Build history of the part. All positions in model axes, mm. Face numbers are marked on the shaded views. A direction names the side the tool comes from. Give positions to 0.01 mm unless a question says otherwise; leave off trailing zeros. Loops run counter-clockwise (first coordinate to the right, second up) from the corner with the lowest first, then second, coordinate; pieces in that order, holes last. Notation, with made-up numbers: (83.25, -5.5) -> (97.25, -5.5) arc R12 ccw to (97.25, -0.5) -> close; hole circle Ø7 at (76.25, 42.25). An arc over 180 degrees is marked (long way). One line per question, with ' | ' between items. Start each with the question number.
(1) Slice it at C-C, the plane y = -28.5. Write the cut outline in (x, z).
(2) Flat gauge pins, fed straight in: pin 1 Ø10 at (x, y) = (15.748, -38.1) entering from -Z; pin 2 Ø12 at (y, z) = (-36, -13.5) entering from -X; pin 3 Ø5 at (x, y) = (110.5, -44) entering from +Z. Where does each tip first touch, or does it go through?
(3) Slice it at D-D, the plane x = 95. Write the cut outline in (y, z).
(4) 3-axis set-ups, long thin cutter, end or side, ignore diameter. For the marked faces 1 and 2: which of +Z, -Z, +X, -X, +Y, -Y reach the whole face in a straight line?
(5) Slice it at A-A, the plane y = -38.1. Write the cut outline in (x, z) (1 decimal).
(6) Drill centre lines: L1, parallel to X at y = -38.1, z = 9.5 (3 decimals); L2, parallel to X at y = -38.1, z = 4.5; L3, parallel to Y at x = 114, z = 4.5. Where is each one in solid material? Low to high. Write a range as from..to.
(7) Slice it at B-B, the plane x = 58. Write the cut outline in (y, z).
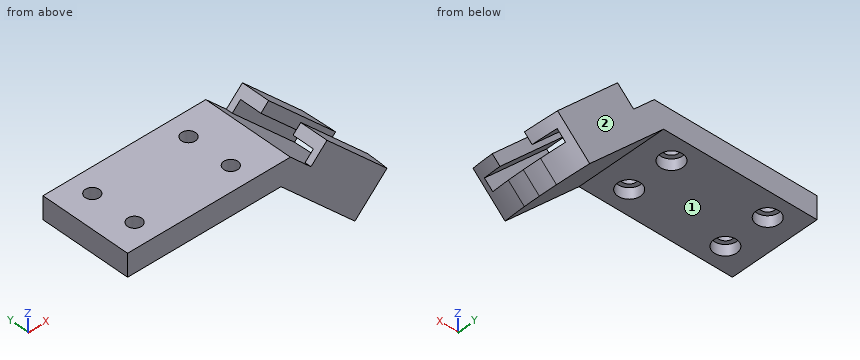
```python
from build123d import *

# Parameters (mm, degrees)
F1_DEPTH       = 50.8
F3_D           = 7.874
F3_CBORE_D     = 12.7
F3_CBORE_DEPTH = 6.096
F4_D           = 7.874
F4_CBORE_D     = 12.7
F4_CBORE_DEPTH = 6.096
F6_DEPTH       = 53.848
F8_DEPTH       = 53.848
F10_DEPTH      = 25.4


with BuildPart() as f1:
    # F0 (on Front) → F1 (new body)
    with BuildSketch(Plane.XZ):
        Polygon((0, 12.7), (0, 0), (85.852, 0), (131.70327, -45.85127), (140.683526, -36.871014), (91.112512, 12.7), align=None)
    extrude(amount=F1_DEPTH)

    # F3 (through all)
    with Locations(Plane(origin=(0, 0, 0), x_dir=(1, 0, 0), z_dir=(0, 0, -1))):
        with Locations((15.748, 38.1)):
            CounterBoreHole(F3_D / 2, F3_CBORE_D / 2, F3_CBORE_DEPTH)

    # F4 (through all)
    with Locations(Plane(origin=(0, 0, 0), x_dir=(1, 0, 0), z_dir=(0, 0, -1))):
        with Locations((69.596, 38.1), (69.596, 12.7), (15.748, 12.7)):
            CounterBoreHole(F4_D / 2, F4_CBORE_D / 2, F4_CBORE_DEPTH)

    # F5 (on face) → F6 (join)
    with BuildSketch(Plane(origin=(88.77727, 0, -88.77727), x_dir=(0, 1, 0), z_dir=(0.707107, 0, -0.707107))):
        Polygon((-3.556, 73.406531), (0, 73.406531), (0, 86.106531), (-15.748, 86.106531), (-15.748, 80.010531), (-3.556, 80.010531), align=None)
    extrude(amount=-F6_DEPTH)

    # F7 (on face) → F8 (join)
    with BuildSketch(Plane(origin=(88.77727, 0, -88.77727), x_dir=(0, 1, 0), z_dir=(0.707107, 0, -0.707107))):
        Polygon((-50.8, 86.106531), (-50.8, 73.406531), (-47.244, 73.406531), (-47.244, 80.010531), (-35.052, 80.010531), (-35.052, 86.106531), align=None)
    extrude(amount=-F8_DEPTH)

    # F9 (on face) → F10 (cut)
    with BuildSketch(Plane(origin=(60.886512, 0, 60.886512), x_dir=(0.707107, 0, -0.707107), z_dir=(0.707107, 0, 0.707107))):
        with BuildLine():
            Line((125.550019, -35.052), (124.677919, -35.052))
            ThreePointArc((124.677919, -35.052), (122.543911, -43.140042), (119.183037, -50.8))
            Line((119.183037, -50.8), (125.550019, -50.8))
            Line((125.550019, -50.8), (125.550019, -35.052))
        make_face()
        with BuildLine():
            ThreePointArc((124.677919, -15.748), (125.331551, -20.554341), (125.550019, -25.4))
            Line((125.550019, -25.4), (125.550019, -15.748))
            Line((125.550019, -15.748), (124.677919, -15.748))
        make_face()
        with BuildLine():
            Line((125.550019, -35.052), (125.550019, -25.4))
            ThreePointArc((125.550019, -25.4), (125.331551, -30.245659), (124.677919, -35.052))
            Line((124.677919, -35.052), (125.550019, -35.052))
        make_face()
        with BuildLine():
            ThreePointArc((119.183037, 0), (122.543911, -7.659958), (124.677919, -15.748))
            Line((124.677919, -15.748), (125.550019, -15.748))
            Line((125.550019, -15.748), (125.550019, 0))
            Line((125.550019, 0), (119.183037, 0))
        make_face()
    extrude(amount=-F10_DEPTH, mode=Mode.SUBTRACT)


solid = f1.part
```
Final values:
1) outline: (0, 0) -> (85.85, 0) -> (131.64, -45.79) -> (140.62, -36.81) -> (91.11, 12.7) -> (0, 12.7) -> close
2) pin 1: z = 6.1 | pin 2: x = 93.35 | pin 3: z = 10.19
3) outline: (-50.8, -9.15) -> (0, -9.15) -> (0, 8.81) -> (-50.8, 8.81) -> close
4) face 1: -Z, -X, +Y, -Y | face 2: +Z, -Z, +X, -X, +Y
5) outline: (0, 0) -> (9.4, 0) -> (9.4, 6.1) -> (11.8, 6.1) -> (11.8, 12.7) -> (0, 12.7) -> close; (19.7, 6.1) -> (22.1, 6.1) -> (22.1, 0) -> (63.2, 0) -> (63.2, 6.1) -> (65.7, 6.1) -> (65.7, 12.7) -> (19.7, 12.7) -> close; (73.5, 6.1) -> (75.9, 6.1) -> (75.9, 0) -> (85.9, 0) -> (130.6, -44.8) -> (139.6, -35.8) -> (91.1, 12.7) -> (73.5, 12.7) -> close; (107.3, 5.9) -> (144.3, -31.1) -> (148.6, -26.8) -> (111.6, 10.2) -> close
6) L1: 0..11.811, 19.685..65.659, 73.533..94.313, 110.902..112.273 | L2: 0..9.4, 22.1..63.25, 75.95..99.31, 108.65..117.27 | L3: -50.8..-35.05, -15.75..0
7) outline: (-50.8, 0) -> (0, 0) -> (0, 12.7) -> (-50.8, 12.7) -> close
